from build123d import *

# Parameters (mm, degrees)
SKETCH1_W           = 154
SKETCH1_H           = 154
SKETCH1_R           = 6.5
BOSS_EXTRUDE1_DEPTH = 10


with BuildPart() as part:
    # Sketch1 → Boss-Extrude1 (new body, symmetric)
    with BuildSketch(Plane.XY):
        Rectangle(SKETCH1_W, SKETCH1_H)
        with Locations((-61, 61)):
            Circle(SKETCH1_R, mode=Mode.SUBTRACT)
        with Locations((61, 61)):
            Circle(SKETCH1_R, mode=Mode.SUBTRACT)
        with Locations((-61, -61)):
            Circle(SKETCH1_R, mode=Mode.SUBTRACT)
        with Locations((61, -61)):
            Circle(SKETCH1_R, mode=Mode.SUBTRACT)
    extrude(amount=BOSS_EXTRUDE1_DEPTH, both=True)


solid = part.part
Could you check a few things on this model? Use its own coordinates, in mm. Give positions to 0.01 mm unless a question says otherwise; leave off trailing zeros. Order: outer loops, then holes, each group sorted by start corner. A loop starts at its lowest first (then second) coordinate and runs counter-clockwise, first axis right, second up. Notation, with made-up numbers: (86, 29.5) - (102, 29.5) arc R14 ccw to (102, 55.5) - close; hole circle Ø6 at (10.25, 0.25). An arc over 180 degrees is marked (long way). Return JSON: item names as keys, results as strings. Group by question number.
Q1. Suppose I cut it at A-A, the plane x = -61. Please give me the cut outline in (y, z), and give its area (3 significant figures).
Q2. Thinking about a two-plate mould opening in Y: for faces 1 (the face through (-58.001, -66.767, -0.14)), 2 (the face through (-1, 1, -10)), 3 (the face through (63.999, 55.233, -0.14)), 4 (the face through (-1, 77, 0)), which applies, pulls with the +Y half, pulls with the -Y half, needs draft (parallel to the pull), parting line crosses it, or undercut?
Q3. Please list where these lines run through material, in increasing order: line 1 along Y through (x, z) = (-61, 2.25); line 2 along X through (y, z) = (-58, -7.5); line 3 along X through (y, z) = (66, -7.75). Write a range as [from, to].
Q4. Suppose I cut it at C-C, the plane z = 7. Please give me the cut outline in (x, y).
Resolved:
{
 "1": {"outline": "(-77, -10) - (-67.5, -10) - (-67.5, 10) - (-77, 10) - close; (-54.5, -10) - (54.5, -10) - (54.5, 10) - (-54.5, 10) - close; (67.5, -10) - (77, -10) - (77, 10) - (67.5, 10) - close", "area": "2,560 mm2"},
 "2": {"face 1": "undercut", "face 2": "needs draft", "face 3": "undercut", "face 4": "pulls with the +Y half"},
 "3": {"line 1": "y = [-77, -67.5], [-54.5, 54.5], [67.5, 77]", "line 2": "x = [-77, -66.77], [-55.23, 55.23], [66.77, 77]", "line 3": "x = [-77, -65.15], [-56.85, 56.85], [65.15, 77]"},
 "4": {"outline": "(-77, -77) - (77, -77) - (77, 77) - (-77, 77) - close; hole circle Ø13 at (-61, -61); hole circle Ø13 at (-61, 61); hole circle Ø13 at (61, -61); hole circle Ø13 at (61, 61)"}
}
